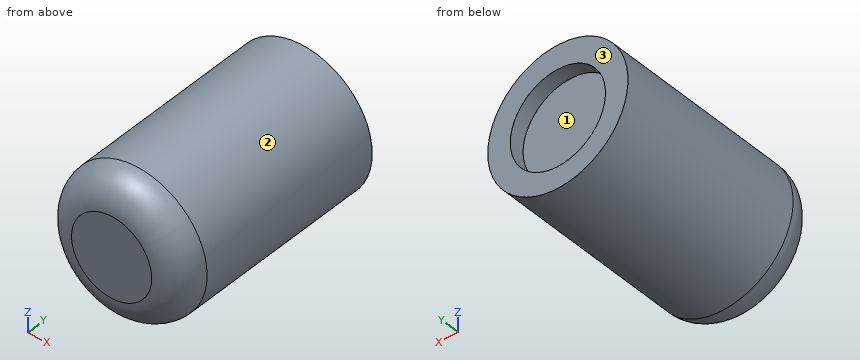
from build123d import *

# Parameters (mm, degrees)
SKETCH_1_R          = 2.8
EXTRUDE_1_DEPTH     = 9
SKETCH_2_R          = 1.9
CUT_EXTRUDE_1_DEPTH = 0.6
FILLET_1_R          = 1.2


with BuildPart() as part:
    # Эскиз1 → Бобышка-Вытянуть1 (new body)
    with BuildSketch(Plane(origin=(0, 0, 0), x_dir=(1, 0, 0), z_dir=(0, 1, 0))):
        Circle(SKETCH_1_R)
    extrude(amount=EXTRUDE_1_DEPTH)

    # Эскиз2 → Вырез-Вытянуть1 (cut)
    with BuildSketch(Plane(origin=(0, 9, 0), x_dir=(1, 0, 0), z_dir=(0, 1, 0))):
        with Locations((0, 0.047154172)):
            Circle(SKETCH_2_R)
    extrude(amount=-CUT_EXTRUDE_1_DEPTH, mode=Mode.SUBTRACT)

    # Скругление1
    fillet_1_edges = [part.edges().sort_by_distance(p)[0] for p in [
        (-2.8, 0, 0),
    ]]
    fillet(fillet_1_edges, radius=FILLET_1_R)


solid = part.part
Design review of the part built by this model. Coordinates are the model's own, in mm. Face numbers are marked on the shaded views. Coordinates: 2 decimals unless noted, no trailing zeros. Order: outer loops, then holes, each group sorted by start corner. A loop starts at its lowest first (then second) coordinate and runs counter-clockwise, first axis right, second up.
Item 1: The part is to be moulded in two halves that separate along Z. For the marked faces 1, 2 and 3, say which applies: pulls with the +Z half, pulls with the -Z half, needs draft (parallel to the pull), parting line crosses it, or undercut.
Item 2: For line 1 (Z direction, x = 0, y = 8.5); line 2 (Y direction, x = -1.55, z = -0.4); line 3 (X direction, y = 0.75, z = 1.65), list the stretches that pass through material, from the lowest coordinate up.
Item 3: Take a section at A-A, the plane x = 0. Write out the cut boundary in (y, z).
Item 4: For pin 1 Ø1 at (y, z) = (7, -2) entering from -X; pin 2 Ø1 at (y, z) = (6.5, 2) entering from +X; pin 3 Ø1.1 at (x, z) = (0, 0.5) entering from +Y, all flat-tipped, find the tip position at first contact; note any pin that passes through.
Item 5: Take a section at B-B, the plane y = 3.75. Write out the cut boundary in (x, z), then the cut area to 3 significant figures.
The answers:
1. face 1: undercut
1. face 2: parting line crosses it
1. face 3: needs draft
2. line 1: z = -2.8 to -1.95, 1.85 to 2.8
2. line 2: y = 0 to 8.4
2. line 3: x = -2.15 to 2.15
3. outline: (0, -1.6) arc R1.2 ccw to (1.2, -2.8) - (9, -2.8) - (9, -1.95) - (8.4, -1.95) - (8.4, 1.85) - (9, 1.85) - (9, 2.8) - (1.2, 2.8) arc R1.2 ccw to (0, 1.6) - close
4. pin 1: stops at x = -2.36
4. pin 2: stops at x = 2.36
4. pin 3: stops at y = 8.4
5. outline: circle Ø5.6 at (0, 0)
5. area: 24.6 mm2
